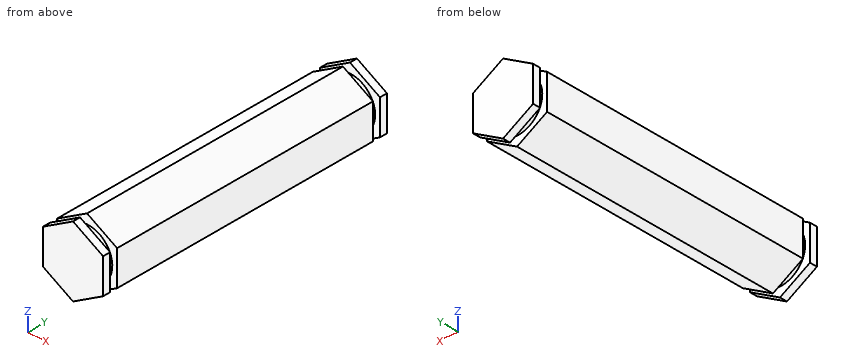
Autodesk Inventor part; units mm, degrees
ref_plane "YZ Plane" through (0, 0, 0) normal (1, 0, 0) x (0, 1, 0)
ref_plane "XZ Plane" through (0, 0, 0) normal (0, 1, 0) x (-1, 0, 0)
ref_plane "XY Plane" through (0, 0, 0) normal (0, 0, 1) x (1, 0, 0)
sketch "Sketch1" plane through (0, 0, 0) normal (0, 1, 0) x (-1, 0, 0)
  line L0 (4.7625, 2.7496) -> (4.7625, -2.7496)
  line L1 (4.7625, -2.7496) -> (0, -5.4993)
  line L2 (0, -5.4993) -> (-4.7625, -2.7496)
  line L3 (-4.7625, -2.7496) -> (-4.7625, 2.7496)
  line L4 (-4.7625, 2.7496) -> (0, 5.4993)
  line L5 (0, 5.4993) -> (4.7625, 2.7496)
  point P0 (0, 0)
  point P1 (0, 0)
  dimension "d0" = 9.525
extrude "Extrusion1" add sketch "Sketch1" along normal blind 49.8
sketch "Sketch2" plane through (0, 0, 0) normal (1, 0, 0) x (0, 1, 0)
  line L0 (1.2, 14) -> (2.4, 14)
  line L1 (2.4, 14) -> (2.4, 4)
  line L2 (2.4, 4) -> (1.2, 4)
  line L3 (1.2, 4) -> (1.2, 14)
  line L4 (0, -2.7496) -> (0, 2.7496)
  line L5 (-9.48, 0) -> (56.88, 0)
  line L6 (47.4, 14) -> (46.2, 14)
  line L7 (46.2, 14) -> (46.2, 4)
  line L8 (46.2, 4) -> (47.4, 4)
  line L9 (47.4, 4) -> (47.4, 14)
  point P0 (0, 0)
  point P1 (0, 0)
  point P2 (1.8, 14)
  dimension "d3" = 1.2
  dimension "d4" = 1.2
  dimension "d5" = 4
  dimension "d6" = 10
  dimension "d8" = 43.8
revolve "Revolution1" cut sketch "Sketch2" angle 360 about axis through (0, -10, 0) along (0, 1, 0)
sketch "Sketch3" plane through (0, 49.8, 0) normal (0, 1, 0) x (1, 0, 0)
  line L0 (0, -5.4993) -> (4.7625, -2.7496)
  line L1 (4.7625, -2.7496) -> (4.7625, 2.7496)
  line L2 (4.7625, 2.7496) -> (0, 5.4993)
  line L3 (0, 5.4993) -> (-4.7625, 2.7496)
  line L4 (-4.7625, 2.7496) -> (-4.7625, -2.7496)
  line L5 (-4.7625, -2.7496) -> (0, -5.4993)
  point P0 (0, 0)
extrude "Extrusion2" cut sketch "Sketch3" against normal blind 1.2
properties part number "Wasp Intermediate Axel"
For this review, take the finished solid that the model builds, in its own axes (mm). Round coordinates to 2 decimals unless told otherwise and drop trailing zeros. Write each loop counter-clockwise with the first axis right and the second up, starting at its lowest first coordinate (ties: lowest second). Pieces come first, ordered by that corner, then holes.
1) Insertion check: pin 1 Ø1 at (x, y) = (1.5, 35) entering from -Z; pin 2 Ø1.5 at (y, z) = (38.5, -4) entering from +X; pin 3 Ø1 at (x, y) = (2.5, 41.5) entering from +Z. Each pin has a flat end and moves straight along its axis. Give the tip position at first contact, or say it passes through.
Answer below:
pin 1: stops at z = -4.92
pin 2: stops at x = 3.9
pin 3: stops at z = 4.34
2) Take a section at B-B on x = -1.5. Give the boundary of the cut face in (y, z).
Answer below:
outline: (0, -4.63) - (1.2, -4.63) - (1.2, -3.71) - (2.4, -3.71) - (2.4, -4.63) - (46.2, -4.63) - (46.2, -3.71) - (47.4, -3.71) - (47.4, -4.63) - (48.6, -4.63) - (48.6, 4.63) - (47.4, 4.63) - (47.4, 3.71) - (46.2, 3.71) - (46.2, 4.63) - (2.4, 4.63) - (2.4, 3.71) - (1.2, 3.71) - (1.2, 4.63) - (0, 4.63) - close
3) For line 1 along Y through (x, z) = (-3.5, 2); line 2 along Z through (x, y) = (1.5, 26.5); line 3 along X through (y, z) = (38, -3), list the stretches that pass through material, from the lowest coordinate up.
Answer below:
line 1: y = 0 to 1.2, 2.4 to 46.2, 47.4 to 48.6
line 2: z = -4.63 to 4.63
line 3: x = -4.33 to 4.33
4) Take a section at A-A on y = 37. Give the boundary of the cut face in (x, z), then the cut area to 3 significant figures.
Answer below:
outline: (-4.76, -2.75) - (0, -5.5) - (4.76, -2.75) - (4.76, 2.75) - (0, 5.5) - (-4.76, 2.75) - close
area: 78.6 mm2
5) Take a section at C-C on z = 2.25. Give the boundary of the cut face in (x, y), then the cut area to 3 significant figures.
Answer below:
outline: (-4.76, 0) - (4.76, 0) - (4.76, 1.2) - (3.31, 1.2) - (3.31, 2.4) - (4.76, 2.4) - (4.76, 46.2) - (3.31, 46.2) - (3.31, 47.4) - (4.76, 47.4) - (4.76, 48.6) - (-4.76, 48.6) - (-4.76, 47.4) - (-3.31, 47.4) - (-3.31, 46.2) - (-4.76, 46.2) - (-4.76, 2.4) - (-3.31, 2.4) - (-3.31, 1.2) - (-4.76, 1.2) - close
area: 456 mm2
